from build123d import *

# Parameters (mm, degrees)
ESQUISSE1_R                                       = 1.65
BOSS_EXTRU_1_DEPTH                                = 2
BOSS_EXTRU_2_DEPTH                                = 48
BOSS_EXTRU_3_DEPTH                                = 3
CONG_1_R                                          = 6
ESQUISSE6_W                                       = 52
ESQUISSE6_H                                       = 8
BOSS_EXTRU_4_DEPTH                                = 20
BOSS_EXTRU_5_DEPTH                                = 8
ESQUISSE8_W                                       = 32.5
ESQUISSE8_H                                       = 11
BOSS_EXTRU_7_DEPTH                                = 3
FRAISAGE_POUR_VIS_T_TE_FRAIS_E_M51_AT_COUNT       = 2
FRAISAGE_POUR_VIS_T_TE_FRAIS_E_M51_AT_PITCH       = 57.584720196
FRAISAGE_POUR_VIS_T_TE_FRAIS_E_M51_2_COUNT        = 2
FRAISAGE_POUR_VIS_T_TE_FRAIS_E_M51_2_PITCH        = 74.276510419
FRAISAGE_POUR_VIS_T_TE_FRAIS_E_M51_3_COUNT        = 2
FRAISAGE_POUR_VIS_T_TE_FRAIS_E_M51_3_PITCH        = 34
FRAISAGE_POUR_VIS_T_TE_FRAIS_E_M51_4_COUNT        = 2
FRAISAGE_POUR_VIS_T_TE_FRAIS_E_M51_4_PITCH        = 63.239623655
CONG_3_R                                          = 6
CONG_4_R                                          = 6
CHAMBRAGE_POUR_VIS_SIX_PANS_CREUX_M31_D           = 3.4
CHAMBRAGE_POUR_VIS_SIX_PANS_CREUX_M31_CBORE_D     = 6.5
CHAMBRAGE_POUR_VIS_SIX_PANS_CREUX_M31_CBORE_DEPTH = 3.4


with BuildPart() as part:
    # Esquisse1 → Boss.-Extru.1 (new, symmetric)
    with BuildSketch(Plane.XY):
        with BuildLine():
            Line((-11.5, 0), (-11.5, 21.5))
            Line((-11.5, 21.5), (-24.5, 21.5))
            Line((-24.5, 21.5), (-24.5, -24.5))
            Line((-24.5, -24.5), (24.5, -24.5))
            Line((24.5, -24.5), (24.5, 21.5))
            Line((24.5, 21.5), (11.5, 21.5))
            Line((11.5, 21.5), (11.5, 0))
            ThreePointArc((11.5, 0), (0, -11.5), (-11.5, 0))
        make_face()
        with Locations((-15.5, 15.5)):
            Circle(ESQUISSE1_R, mode=Mode.SUBTRACT)
        with Locations((15.5, 15.5)):
            Circle(ESQUISSE1_R, mode=Mode.SUBTRACT)
        with Locations((15.5, -15.5)):
            Circle(ESQUISSE1_R, mode=Mode.SUBTRACT)
        with Locations((-15.5, -15.5)):
            Circle(ESQUISSE1_R, mode=Mode.SUBTRACT)
    extrude(amount=BOSS_EXTRU_1_DEPTH, both=True)

    # Esquisse2 → Boss.-Extru.2 (add)
    with BuildSketch(Plane(origin=(0, 0, -2), x_dir=(-1, 0, 0), z_dir=(0, 0, -1))):
        Polygon((-24.5, 21.5), (-21.5, 21.5), (-21.5, -21.5), (21.5, -21.5), (21.5, 21.5), (24.5, 21.5), (24.5, -24.5), (-24.5, -24.5), align=None)
    extrude(amount=BOSS_EXTRU_2_DEPTH)

    # Esquisse4 → Boss.-Extru.3 (add)
    with BuildSketch(Plane(origin=(0, 0, -50), x_dir=(-1, 0, 0), z_dir=(0, 0, -1))):
        with BuildLine():
            Line((-24.5, 21.5), (-44.5, 21.5))
            Line((-44.5, 21.5), (-44.5, -24.5))
            ThreePointArc((-44.5, -24.5), (-38.642135624, -38.642135624), (-24.5, -44.5))
            Line((-24.5, -44.5), (24.5, -44.5))
            Line((24.5, -44.5), (24.5, -24.5))
            Line((24.5, -24.5), (-24.5, -24.5))
            Line((-24.5, -24.5), (-24.5, 21.5))
        make_face()
    extrude(amount=-BOSS_EXTRU_3_DEPTH)

    # Congé1
    cong_1_edges = [part.edges().sort_by_distance(p)[0] for p in [
        (0, -21.5, -50),
        (21.5, 0, -50),
        (24.5, -1.5, -47),
        (0, -24.5, -47),
    ]]
    fillet(cong_1_edges, radius=CONG_1_R)

    # Esquisse6 → Boss.-Extru.4 (add)
    with BuildSketch(Plane.ZY.offset(24.5)):
        with Locations((-24, 14.5)):
            Rectangle(ESQUISSE6_W, ESQUISSE6_H)
    extrude(amount=BOSS_EXTRU_4_DEPTH)

    # Esquisse7 → Boss.-Extru.5 (add)
    with BuildSketch(Plane(origin=(0, 18.5, 0), x_dir=(1, 0, 0), z_dir=(0, 1, 0))):
        Polygon((-44.5, -2), (-44.5, -30), (-35.5, -30), (-24.5, -2), align=None)
    extrude(amount=-BOSS_EXTRU_5_DEPTH)

    # Esquisse8 → Boss.-Extru.7 (add)
    with BuildSketch(Plane(origin=(0, 0, -50), x_dir=(-1, 0, 0), z_dir=(0, 0, -1))):
        with Locations((40.75, 16)):
            Rectangle(ESQUISSE8_W, ESQUISSE8_H)
    extrude(amount=-BOSS_EXTRU_7_DEPTH)

    # Esquisse5 → Fraisage pour vis à tête fraisée M51 (revolve, cut)
    with BuildSketch(Plane(origin=(-17, -37, -47), x_dir=(0, -1, 0), z_dir=(1, 0, 0))):
        Polygon((0, 0), (0, 3), (2.75, 3), (2.75, 2.45), (5.2, 0), align=None)
    fraisage_pour_vis_t_te_frais_e_m51 = revolve(axis=Axis((-17, -37, -40.65), (0, 0, -1)), mode=Mode.SUBTRACT)

    # Fraisage pour vis à tête fraisée M51 at: Fraisage pour vis à tête fraisée M51 ×2
    with Locations(*[Vector(0.9377487607237037, 0.3473143558235938, 0) * (i * FRAISAGE_POUR_VIS_T_TE_FRAIS_E_M51_AT_PITCH) for i in range(1, FRAISAGE_POUR_VIS_T_TE_FRAIS_E_M51_AT_COUNT)]):
        add(fraisage_pour_vis_t_te_frais_e_m51, mode=Mode.SUBTRACT)

    # Fraisage pour vis _ t_te frais_e M51 2: Fraisage pour vis à tête fraisée M51 ×2
    with Locations(*[Vector(0.7270131525498176, 0.6866235329637164, 0) * (i * FRAISAGE_POUR_VIS_T_TE_FRAIS_E_M51_2_PITCH) for i in range(1, FRAISAGE_POUR_VIS_T_TE_FRAIS_E_M51_2_COUNT)]):
        add(fraisage_pour_vis_t_te_frais_e_m51, mode=Mode.SUBTRACT)

    # Fraisage pour vis _ t_te frais_e M51 3: Fraisage pour vis à tête fraisée M51 ×2
    with Locations(*[(i * FRAISAGE_POUR_VIS_T_TE_FRAIS_E_M51_3_PITCH, 0, 0) for i in range(1, FRAISAGE_POUR_VIS_T_TE_FRAIS_E_M51_3_COUNT)]):
        add(fraisage_pour_vis_t_te_frais_e_m51, mode=Mode.SUBTRACT)

    # Fraisage pour vis _ t_te frais_e M51 4: Fraisage pour vis à tête fraisée M51 ×2
    with Locations(*[Vector(-0.5455440435307616, 0.8380821538298656, 0) * (i * FRAISAGE_POUR_VIS_T_TE_FRAIS_E_M51_4_PITCH) for i in range(1, FRAISAGE_POUR_VIS_T_TE_FRAIS_E_M51_4_COUNT)]):
        add(fraisage_pour_vis_t_te_frais_e_m51, mode=Mode.SUBTRACT)

    # Congé3
    # the kernel refuses this fillet: 6 mm, written as the material it adds along each edge
    with BuildSketch(Plane(origin=(-44.5, 18.5, -47), x_dir=(0, 0, 1), z_dir=(1, 0, 0))) as cong_3_piece_1_section:
        with BuildLine():
            CenterArc((5.196152423, -6), CONG_3_R, 90, 60)
            Line((0, -3), (0, 0))
            Line((0, 0), (5.196152423, 0))
        make_face()
    cong_3_piece_1 = extrude(amount=32.990381057, mode=Mode.PRIVATE)
    cong_3_piece_1 = split(cong_3_piece_1, bisect_by=Plane(origin=(-21.5, 18.653513823, -43.204827013), z_dir=(-1, 0, 0)), keep=Keep.TOP, mode=Mode.PRIVATE)
    add(cong_3_piece_1)
    with BuildSketch(Plane(origin=(-24.5, 18.5, -47), x_dir=(0, 0, 1), z_dir=(0, 1, 0))) as cong_3_piece_2:
        with BuildLine():
            CenterArc((CONG_3_R, -CONG_3_R), CONG_3_R, 90, 90)
            Line((0, -CONG_3_R), (0, 0))
            Line((0, 0), (CONG_3_R, 0))
        make_face()
    extrude(amount=3)

    # Congé4
    cong_4_edges = [part.edges().sort_by_distance(p)[0] for p in [
        (-24.5, 14.5, 2),
    ]]
    fillet(cong_4_edges, radius=CONG_4_R)

    # Chambrage pour vis à six pans creux M31 (through all)
    with Locations(Plane(origin=(-40, 18.5, -20), x_dir=(0, 0, 1), z_dir=(0, 1, 0))):
        with Locations((0, 0), (20, 0), (40, 0)):
            CounterBoreHole(CHAMBRAGE_POUR_VIS_SIX_PANS_CREUX_M31_D / 2, CHAMBRAGE_POUR_VIS_SIX_PANS_CREUX_M31_CBORE_D / 2, CHAMBRAGE_POUR_VIS_SIX_PANS_CREUX_M31_CBORE_DEPTH)


solid = part.part
Could you check a few things on this model? Use its own coordinates, in mm. A direction names the side the tool comes from. Give positions to 0.01 mm unless a question says otherwise; leave off trailing zeros. Loops run counter-clockwise (first coordinate to the right, second up) from the corner with the lowest first, then second, coordinate; pieces in that order, holes last. Notation, with made-up numbers: (88, -1) -> (94, -1) arc R13 ccw to (94, 17) -> close; hole circle Ø6 at (58.5, 87.5). An arc over 180 degrees is marked (long way). Answer as CSV lines item,"result". Start each with the question number.
(1) I'm going to push flat-ended pins straight in: pin 1 Ø7 at (x, z) = (-40.5, 21) entering from +Y; pin 2 Ø13 at (x, z) = (0, -20) entering from -Y; pin 3 Ø7 at (x, y) = (-17, -37) entering from +Z; pin 4 Ø2 at (x, y) = (15.5, 15.5) entering from -Z. Where does each tip first touch, or does it pass through?
(2) I need wall thicknesses on probe 1 along Y at (x, z) = (-15.5, -0.3); probe 2 along X at (y, z) = (-1, -37); probe 3 along Z at (x, y) = (-4, -14.5). Which ranges of each line are inside material? Lowest first, please.
(3) If we section it at B-B on z = -20: Write out the boundary of the cut face in (x, y), then the cut area to 3 significant figures.
(4) Which directions (+Z, -Z, +X, -X, +Y, -Y) give clear straight access to the entire face, cutting with the end or side of a thin tool? Please do faces 4 (the flat face through (-41.4, 15.1, 21.4)), 5 (the flat face through (0, -24.5, -19)), 6 (the flat face through (11.5, 11, 0)), 7 (the flat face through (0, -14, -2)).
(5) If we section it at D-D on y = -4: Write out the boundary of the cut face in (x, z), then the cut area to 3 significant figures.
(6) If we section it at A-A on x = 37: Write out the boundary of the cut face in (y, z).
(7) We'd pull the mould along X, two halves only. Please class faces 1 (the conical face through (-15.89, -39.68, -49.3)), 2 (the flat face through (31, -24, -47)), 3 (the cylindrical face through (38.797, -38.486, -48.521)): released by +X, released by -X, zero draft, split by the parting line, or undercut.
(8) If we section it at C-C on y = -37: Write out the boundary of the cut face in (x, z), then the cut area to 3 significant figures.
Computed:
1,pin 1,"stops at y = 18.5"
1,pin 2,"stops at y = -24.5"
1,pin 3,"stops at z = -48.7"
1,pin 4,"passes through"
2,probe 1,"y = -24.5 to -17.15, -13.85 to 13.85, 17.15 to 21.5"
2,probe 2,"x = -24.5 to -21.5, 21.5 to 24.5"
2,probe 3,"z = -2 to 2"
3,outline,"(-44.5, 10.5) -> (-41.7, 10.5) -> (-41.7, 15.1) -> (-43.25, 15.1) -> (-43.25, 18.5) -> (-44.5, 18.5) -> close; (-38.3, 10.5) -> (-24.5, 10.5) -> (-24.5, -24.5) -> (24.5, -24.5) -> (24.5, 21.5) -> (21.5, 21.5) -> (21.5, -21.5) -> (-21.5, -21.5) -> (-21.5, 21.5) -> (-24.5, 21.5) -> (-24.5, 18.5) -> (-36.75, 18.5) -> (-36.75, 15.1) -> (-38.3, 15.1) -> close"
3,area,"527 mm2"
4,face 4,"+Y"
4,face 5,"+Z, +X, -X, -Y"
4,face 6,"+Z, -Z, +Y"
4,face 7,"-Z, +Y"
5,outline,"(-24.5, -50) -> (-21.5, -50) -> (-21.5, -2) -> (-10.78, -2) -> (-10.78, 2) -> (-24.5, 2) -> close; (10.78, -2) -> (21.5, -2) -> (21.5, -44) arc R6 ccw to (27.5, -50) -> (44.5, -50) -> (44.5, -47) -> (30.5, -47) arc R6 cw to (24.5, -41) -> (24.5, 2) -> (10.78, 2) -> close"
5,area,"458 mm2"
6,outline,"(-40.11, -50) -> (-19.75, -50) -> (-19.75, -49.45) -> (-22.2, -47) -> (-40.11, -47) -> close; (-14.25, -50) -> (11.25, -50) -> (11.25, -49.45) -> (8.8, -47) -> (-11.8, -47) -> (-14.25, -49.45) -> close; (16.75, -50) -> (21.5, -50) -> (21.5, -47) -> (19.2, -47) -> (16.75, -49.45) -> close"
7,face 1,"undercut"
7,face 2,"zero draft"
7,face 3,"released by +X"
8,outline,"(-24.5, -50) -> (-19.75, -50) -> (-19.75, -49.45) -> (-22.2, -47) -> (-24.5, -47) -> close; (-14.25, -50) -> (14.25, -50) -> (14.25, -49.45) -> (11.8, -47) -> (-11.8, -47) -> (-14.25, -49.45) -> close; (19.75, -50) -> (40.11, -50) -> (40.11, -47) -> (22.2, -47) -> (19.75, -49.45) -> close"
8,area,"149 mm2"
